Can you work these out from the model? Positions are in its coordinate system, mm. Coordinates: 2 decimals unless noted, no trailing zeros. Order: outer loops, then holes, each group sorted by start corner. A loop starts at its lowest first (then second) coordinate and runs counter-clockwise, first axis right, second up. Notation, with made-up numbers: M 60,27 L 81,27 A23 cw 81,42 Z; hole C 20,8 d10. An arc over 180 degrees is marked long. Answer as CSV lines item,"result". Start each with the question number.
1. I need wall thicknesses on line 1 along X through (y, z) = (-4.3, -35); line 2 along X through (y, z) = (-3.15, -15); line 3 along Z through (x, y) = (9, -5.45). Which ranges of each line are inside material? Lowest first, please. Write a range as from..to.
2. If we section it at D-D (x = 17): List the corners of the cut face in (y, z) for me, plus the area to 3 significant figures.
3. If we section it at A-A (z = -15): List the corners of the cut face in (x, y) for me.
4. If we mould it in two halves opening along Z, with no side actions, what happens to faces 1 (the face through (17.237, -2.958, -91.773)), 2 (the face through (10, -3, -27)), 3 (the face through (50, -3, -100)), 4 (the face through (49, -3, 0))? For each: released by +Z, released by -Z, zero draft, split by the parting line, or undercut.
5. If we section it at C-C (x = 95): List the corners of the cut face in (y, z) for me, plus the area to 3 significant figures.
6. If we section it at B-B (y = -2.7): Give the number of separate pieces and of enclosed holes in the cut face, plus the area to 3 significant figures.
7. Will these pins go through, and if not, where does the flat tip stop? pin 1 (1 mm diameter, centred on x = 67, z = -86.5, fed in from +Y); pin 2 (1 mm diameter, centred on y = -4, z = -77.5, fed in from +X).
```python
from build123d import *

# Parameters (mm, degrees)
DODANIE_WYCI_GNI_CIE1_DEPTH = 6
SZKIC2_R                    = 5.4
WYTNIJ_WYCI_GNI_CIE1_DEPTH  = 142.548578234
SZKIC3_R                    = 1.55
WYTNIJ_WYCI_GNI_CIE2_DEPTH  = 142.548578234
SZKIC4_R                    = 3
WYTNIJ_WYCI_GNI_CIE3_DEPTH  = 142.548578234


with BuildPart() as part:
    # Szkic1 → Dodanie-wyciągnięcie1 (new body)
    with BuildSketch(Plane(origin=(0, 0, 0), x_dir=(1, 0, 0), z_dir=(0, 1, 0))):
        with BuildLine():
            Line((10, 0), (90, 0))
            ThreePointArc((90, 0), (97.071067812, 2.928932188), (100, 10))
            Line((100, 10), (100, 75))
            ThreePointArc((100, 75), (92.67766953, 92.67766953), (75, 100))
            Line((75, 100), (25, 100))
            ThreePointArc((25, 100), (7.32233047, 92.67766953), (0, 75))
            Line((0, 75), (0, 10))
            ThreePointArc((0, 10), (2.928932188, 2.928932188), (10, 0))
        make_face()
    extrude(amount=-DODANIE_WYCI_GNI_CIE1_DEPTH)

    # Szkic2 → Wytnij-wyciągnięcie1 (cut, through all)
    with BuildSketch(Plane(origin=(0, 0, 0), x_dir=(1, 0, 0), z_dir=(0, 1, 0))):
        with Locations(Location((17, 86.378345537, 0), (0, 0, 270))):
            Circle(SZKIC2_R)
        with Locations(Location((83, 86.378345537, 0), (0, 0, 270))):
            Circle(SZKIC2_R)
        with Locations(Location((15, 15, 0), (0, 0, 270))):
            Circle(SZKIC2_R)
        with Locations(Location((85, 15, 0), (0, 0, 270))):
            Circle(SZKIC2_R)
    extrude(amount=-WYTNIJ_WYCI_GNI_CIE1_DEPTH, mode=Mode.SUBTRACT)

    # Szkic3 → Wytnij-wyciągnięcie2 (cut, through all)
    with BuildSketch(Plane.XZ.offset(6)):
        with Locations(Location((5, -35, 0), (0, 0, 270))):
            Circle(SZKIC3_R)
        with Locations(Location((95, -35, 0), (0, 0, 270))):
            Circle(SZKIC3_R)
    extrude(amount=-WYTNIJ_WYCI_GNI_CIE2_DEPTH, mode=Mode.SUBTRACT)

    # Szkic4 → Wytnij-wyciągnięcie3 (cut, through all)
    with BuildSketch(Plane(origin=(0, 0, 0), x_dir=(1, 0, 0), z_dir=(0, 1, 0))):
        with Locations(Location((90, 24, 0), (0, 0, 270))):
            Circle(SZKIC4_R)
        with Locations(Location((10, 24, 0), (0, 0, 270))):
            Circle(SZKIC4_R)
    extrude(amount=-WYTNIJ_WYCI_GNI_CIE3_DEPTH, mode=Mode.SUBTRACT)


solid = part.part
```
Solved:
1,line 1,"0..3.45, 6.55..93.45, 96.55..100"
1,line 2,"0..9.6, 20.4..79.6, 90.4..100"
1,line 3,"-94.21..-26.83, -21.17..-0.05"
2,outline,"M -6,-98.69 L 0,-98.69 L 0,-91.78 L -6,-91.78 Z; M -6,-80.98 L 0,-80.98 L 0,-20.02 L -6,-20.02 Z; M -6,-9.98 L 0,-9.98 L 0,0 L -6,0 Z"
2,area,"467 mm²"
3,outline,"M 0,-6 L 9.6,-6 L 9.6,0 L 0,0 Z; M 20.4,-6 L 79.6,-6 L 79.6,0 L 20.4,0 Z; M 90.4,-6 L 100,-6 L 100,0 L 90.4,0 Z"
4,face 1,"undercut"
4,face 2,"undercut"
4,face 3,"released by -Z"
4,face 4,"released by +Z"
5,outline,"M -6,-90 L 0,-90 L 0,-36.55 L -6,-36.55 Z; M -6,-33.45 L 0,-33.45 L 0,-1.34 L -6,-1.34 Z"
5,area,"513 mm²"
6,separate pieces,"1"
6,enclosed holes,"8"
6,area,"9,250 mm²"
7,pin 1,"y = 0"
7,pin 2,"x = 99.92"
